Model file for the job. Use its own axes, mm. A direction names the side the tool comes from. Coordinates: 2 decimals unless noted, no trailing zeros. Order: outer loops, then holes, each group sorted by start corner. A loop starts at its lowest first (then second) coordinate and runs counter-clockwise, first axis right, second up.
from build123d import *

# Parameters (mm, degrees)
BOSS_EXTRUDE1_DEPTH = 18
SKETCH2_R           = 1.75
CUT_EXTRUDE1_DEPTH  = 33.5
CUT_EXTRUDE2_DEPTH  = 1
CUT_EXTRUDE3_DEPTH  = 5


with BuildPart() as part:
    # Sketch1 → Boss-Extrude1 (new body)
    with BuildSketch(Plane(origin=(0, 0, 0), x_dir=(1, 0, 0), z_dir=(0, 1, 0))):
        with BuildLine():
            Line((-11.998275301, 32.528571429), (-29.498275301, 32.528571429))
            Line((-29.498275301, 32.528571429), (-29.498275301, 19.914699304))
            ThreePointArc((-29.498275301, 19.914699304), (-21.114218589, 23.723916882), (-11.998275301, 25.028571429))
            Line((-11.998275301, 25.028571429), (-11.998275301, 32.528571429))
        make_face()
        with BuildLine():
            ThreePointArc((-11.998275301, 25.028571429), (-21.114218589, 23.723916882), (-29.498275301, 19.914699304))
            ThreePointArc((-29.498275301, 19.914699304), (-44.498275301, -7.471428571), (-29.498275301, -34.857556447))
            ThreePointArc((-29.498275301, -34.857556447), (-21.114218589, -38.666774025), (-11.998275301, -39.971428571))
            Line((-11.998275301, -39.971428571), (-11.998275301, -32.971428571))
            ThreePointArc((-11.998275301, -32.971428571), (-37.498275301, -7.471428571), (-11.998275301, 18.028571429))
            Line((-11.998275301, 18.028571429), (-11.998275301, 25.028571429))
        make_face()
        with BuildLine():
            Line((-29.498275301, -34.857556447), (-29.498275301, -47.471428571))
            Line((-29.498275301, -47.471428571), (-11.998275301, -47.471428571))
            Line((-11.998275301, -47.471428571), (-11.998275301, -39.971428571))
            ThreePointArc((-11.998275301, -39.971428571), (-21.114218589, -38.666774025), (-29.498275301, -34.857556447))
        make_face()
    extrude(amount=BOSS_EXTRUDE1_DEPTH)

    # Sketch2 → Cut-Extrude1 (cut, through all)
    with BuildSketch(Plane(origin=(-11.998275301, 0, 0), x_dir=(0, 0, -1), z_dir=(1, 0, 0))):
        with Locations((-42.471428571, 5.25)):
            Circle(SKETCH2_R)
        with Locations((27.528571429, 5.25)):
            Circle(SKETCH2_R)
    extrude(amount=-CUT_EXTRUDE1_DEPTH, mode=Mode.SUBTRACT)

    # Sketch3 → Cut-Extrude2 (cut)
    with BuildSketch(Plane(origin=(-11.998275301, 0, 0), x_dir=(0, 0, -1), z_dir=(1, 0, 0))):
        Polygon((-42.144930844, 15.142571671), (-39.566939391, 15.142571671), (-39.566939391, 14.192785347), (-41.195144519, 14.192785347), (-41.195144519, 13.175157142), (-39.566939391, 13.175157142), (-39.566939391, 12.225370817), (-41.195144519, 12.225370817), (-41.195144519, 9.850905005), (-42.144930844, 9.850905005), align=None)
        Polygon((-38.820678707, 15.142571671), (-35.42858469, 15.142571671), (-35.42858469, 14.64965801), (-37.762769385, 9.715221244), (-38.603372684, 10.139232996), (-36.653978654, 14.260627227), (-38.820678707, 14.260627227), align=None)
    extrude(amount=-CUT_EXTRUDE2_DEPTH, mode=Mode.SUBTRACT)

    # Sketch4 → Cut-Extrude3 (cut)
    with BuildSketch(Plane.ZY.offset(29.498275301)):
        Polygon((45.042020782, 3.385760472), (45.371203467, 6.544078393), (42.800611256, 8.408317922), (39.900836361, 7.114239528), (39.571653676, 3.955921607), (42.142245887, 2.091682078), align=None)
        Polygon((-25.283205831, 3.004634402), (-24.461344982, 6.071860849), (-26.706710579, 8.317226447), (-29.773937026, 7.495365598), (-30.595797876, 4.428139151), (-28.350432278, 2.182773553), align=None)
    extrude(amount=-CUT_EXTRUDE3_DEPTH, mode=Mode.SUBTRACT)


solid = part.part
Q1. Cut at B-B, the plane y = 5.25. List the corners of the cut face in (x, z), plus the area to 3 significant figures.
Established:
outline: (-29.5, -32.53) - (-12, -32.53) - (-12, -29.28) - (-24.5, -29.28) - (-24.5, -30.38) - (-29.5, -30.38) - close; (-29.5, -24.68) - (-24.5, -24.68) - (-24.5, -25.78) - (-12, -25.78) - (-12, -18.03) arc R25.5 cw to (-12, 32.97) - (-12, 40.72) - (-24.5, 40.72) - (-24.5, 39.71) - (-29.5, 39.71) - (-29.5, 34.86) arc R32.5 ccw to (-29.5, -19.91) - close; (-29.5, 45.24) - (-24.5, 45.24) - (-24.5, 44.22) - (-12, 44.22) - (-12, 47.47) - (-29.5, 47.47) - close
area: 814 mm2
Q2. Mould opens along Z. For faces 5 (the face through (-12.491, 12.171, 37.642)), 6 (the face through (-11.998, 9, -25)), 7 (the face through (-24.498, 4, 44)), 8 (the face through (-44.495, 8.874, 7.015)) say: pulls with the +Z half, pulls with the -Z half, needs draft (parallel to the pull), parting line crosses it, or undercut.
Established:
face 5: undercut
face 6: needs draft
face 7: undercut
face 8: parting line crosses it
Q3. Which spindle directions (+Z, -Z, +X, -X, +Y, -Y) get a long thin tool onto all of the face, cutting with end or side? Do faces 1 (the face through (-29.498, 9, 41)), 2 (the face through (-39, 0, 7)), 3 (the face through (-29.498, 9, -26)), 4 (the face through (-27.033, 3.037, 40.839)). Say none if no direction does.
Established:
face 1: +Z, -X, +Y, -Y
face 2: +Z, -Z, +X, -X, -Y
face 3: -Z, -X, +Y, -Y
face 4: -X
Q4. Probe line 1 (X direction, y = 2.25, z = -23); line 2 (Z direction, x = -17, y = 4); line 3 (Z direction, x = -18.5, y = 2.5). List the from-to ranges inside material, lowest first.
Established:
line 1: x = -29.5 to -12
line 2: z = -32.53 to -28.75, -26.3 to -17.53, 32.48 to 41.25, 43.7 to 47.47
line 3: z = -32.53 to -17.19, 32.13 to 47.47
Q5. Cut at D-D, the plane z = -8. List the corners of the cut face in (x, y), plus the area to 3 significant figures.
Established:
outline: (-40.58, 0) - (-32.27, 0) - (-32.27, 18) - (-40.58, 18) - close
area: 150 mm2
Q6. Drop flat-ended pins along their axis: P1, Ø3, axis at y = 4.5, z = -27.5, coming from the -X side; P2, Ø4.5, axis at y = 4, z = 43, coming from the -X side; P3, Ø5, axis at x = -37.5, y = 9.5, coming from the +Z side. Give the stop position or say it passes through.
Established:
P1: stops at x = -24.5
P2: stops at x = -29.5
P3: stops at z = 30.43
Q7. Cut at C-C, the plane x = -23. List the corners of the cut face in (y, z).
Established:
outline: (0, -32.53) - (18, -32.53) - (18, -15.53) - (0, -15.53) - close; (0, 30.48) - (18, 30.48) - (18, 47.47) - (0, 47.47) - close; hole circle Ø3.5 at (5.25, -27.53); hole circle Ø3.5 at (5.25, 42.47)
Q8. Cut at A-A, the plane x = -17. List the corners of the cut face in (y, z).
Established:
outline: (0, -32.53) - (18, -32.53) - (18, -17.53) - (0, -17.53) - close; (0, 32.48) - (18, 32.48) - (18, 47.47) - (0, 47.47) - close; hole circle Ø3.5 at (5.25, -27.53); hole circle Ø3.5 at (5.25, 42.47)
